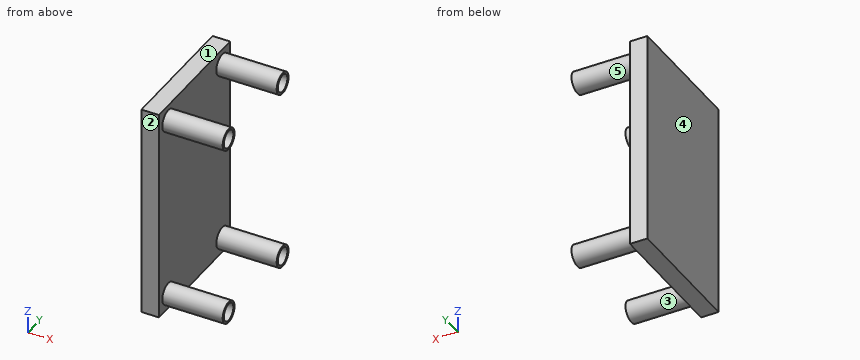
Autodesk Inventor part; units mm, degrees
ref_plane "YZ Plane" through (0, 0, 0) normal (1, 0, 0) x (0, 1, 0)
ref_plane "XZ Plane" through (0, 0, 0) normal (0, 1, 0) x (-1, 0, 0)
ref_plane "XY Plane" through (0, 0, 0) normal (0, 0, 1) x (1, 0, 0)
sketch "スケッチ1" plane through (0, 0, 0) normal (1, 0, 0) x (0, 1, 0)
  line L0 (13.9438, 85.4482) -> (-46.0562, 85.4482)
  line L1 (-46.0562, 85.4482) -> (-46.0562, -14.5518)
  line L2 (-46.0562, -14.5518) -> (13.9438, -14.5518)
  line L3 (13.9438, -14.5518) -> (13.9438, 85.4482)
  point P0 (0, 0)
  dimension "d0" = 60
  dimension "d1" = 100
extrude "押し出し1" add sketch "スケッチ1" along normal blind 8.1
sketch "スケッチ2" plane through (8.1, 0, 0) normal (1, 0, 0) x (0, 0, -1)
  circle A0 centre (-78.096, 7.3739) radius 5
  circle A1 centre (-78.096, -38.2101) radius 5
  circle A2 centre (7.3739, -38.2101) radius 5
  circle A3 centre (7.3739, 7.3739) radius 5
  circle A4 centre (-78.096, 7.3739) radius 4
  circle A5 centre (-78.096, -38.2101) radius 4
  circle A6 centre (7.3739, 7.3739) radius 4
  circle A7 centre (7.3739, -38.2101) radius 4
  point P0 (0, 0)
  dimension "d4" = 10
  dimension "d5" = 10
  dimension "d6" = 10
  dimension "d7" = 10
  dimension "d8" = 8
  dimension "d9" = 8
  dimension "d10" = 8
  dimension "d11" = 8
extrude "押し出し2" add sketch "スケッチ2" along normal blind 28
sketch "スケッチ3" plane through (0, 0, 0) normal (-1, 0, 0) x (0, 0, 1)
  point P0 (0, 0)
equation "\"BendRadius\" = Thickness"
equation "\"BendReliefWidth\" = Thickness"
equation "\"BendReliefDepth\" = 0.5 * Thickness"
equation "\"CornerReliefSize\" = 4 * Thickness"
equation "\"MinimumRemnant\" = 2 * Thickness"
equation "\"TransitionRadius\" = BendRadius"
equation "\"JacobiRadiusSize\" = BendRadius"
equation "\"GapSize\" = Thickness"
For this review, take the finished solid that the model builds, in its own axes (mm). Face numbers are marked on the shaded views. A direction names the side the tool comes from. Coordinates: 2 decimals unless noted, no trailing zeros. Write each loop counter-clockwise with the first axis right and the second up, starting at its lowest first coordinate (ties: lowest second). Pieces come first, ordered by that corner, then holes. Notation, with made-up numbers: (-20.5, 43.25) - (18.5, 43.25) arc R19 cw to (18.5, 56.25) - close; hole circle Ø4 at (23, 27). An arc over 180 degrees is marked (long way). Answer in a Markdown table with one row per item. Add a question column.
Q1. For probe 1 along Y at (x, z) = (33, 78.5); probe 2 along Y at (x, z) = (30, 81); probe 3 along Z at (x, y) = (33.5, -39), list the stretches that pass through material, from the lowest coordinate up.
Q2. We need section C-C, the plane z = -5. State the section outline as (x, y) points, and give its area (3 significant figures).
Q3. Tool access review of the marked faces 4 and 5: name each direction out of +Z, -Z, +X, -X, +Y, -Y from which nothing blocks a thin tool from reaching the whole face with its end or side.
Q4. Draft analysis for pull direction Y (two halves, no side actions). For the marked faces 1, 2 and 3, state which applies: +Y half, -Y half, draft (parallel to the pull), parting line (faces both ways), or undercut.
Q5. We need section D-D, the plane y = -40. State the section outline as (x, z) points.
Q6. We need section B-B, the plane y = -31.5. State the section outline as (x, z) points, and give its area (3 significant figures).
Q7. For P1, Ø1, axis at y = -35, z = 34, coming from the +X side; P2, Ø12, axis at x = 16.5, z = 12.5, coming from the -Y side; P3, Ø12, axis at x = 31.5, z = 3, coming from the +Y side, all flat-tipped, find the tip position at first contact; note any pin that passes through.
Q8. We need section A-A, the plane x = 22. State the section outline as (y, z) points, and give its area (3 significant figures).
Answer list:
| question | item | result |
|---|---|---|
| 1 | probe 1 | y = -43.19 to -42.19, -34.23 to -33.23, 2.39 to 3.39, 11.35 to 12.36 |
| 1 | probe 2 | y = -42.28 to -40.96, -35.46 to -34.14, 3.3 to 4.62, 10.12 to 11.44 |
| 1 | probe 3 | z = -12.31 to -11.3, -3.45 to -2.44, 73.16 to 74.17, 82.02 to 83.03 |
| 2 | outline | (0, -46.06) - (8.1, -46.06) - (8.1, -42.61) - (36.1, -42.61) - (36.1, -41.43) - (8.1, -41.43) - (8.1, -34.99) - (36.1, -34.99) - (36.1, -33.81) - (8.1, -33.81) - (8.1, 2.97) - (36.1, 2.97) - (36.1, 4.15) - (8.1, 4.15) - (8.1, 10.59) - (36.1, 10.59) - (36.1, 11.77) - (8.1, 11.77) - (8.1, 13.94) - (0, 13.94) - close |
| 2 | area | 618 mm2 |
| 3 | face 4 | +Z, -Z, -X, +Y, -Y |
| 3 | face 5 | +X |
| 4 | face 1 | draft |
| 4 | face 2 | -Y half |
| 4 | face 3 | undercut |
| 5 | outline | (0, -14.55) - (8.1, -14.55) - (8.1, -12.04) - (36.1, -12.04) - (36.1, -10.95) - (8.1, -10.95) - (8.1, -3.8) - (36.1, -3.8) - (36.1, -2.71) - (8.1, -2.71) - (8.1, 73.43) - (36.1, 73.43) - (36.1, 74.52) - (8.1, 74.52) - (8.1, 81.67) - (36.1, 81.67) - (36.1, 82.76) - (8.1, 82.76) - (8.1, 85.45) - (0, 85.45) - close |
| 6 | outline | (0, -14.55) - (8.1, -14.55) - (8.1, 85.45) - (0, 85.45) - close |
| 6 | area | 810 mm2 |
| 7 | P1 | stops at x = 8.1 |
| 7 | P2 | passes through |
| 7 | P3 | stops at y = 9.8 |
| 8 | outline | circle Ø10 at (-38.21, -7.37); circle Ø10 at (-38.21, 78.1); circle Ø10 at (7.37, -7.37); circle Ø10 at (7.37, 78.1); hole circle Ø8 at (-38.21, -7.37); hole circle Ø8 at (-38.21, 78.1); hole circle Ø8 at (7.37, -7.37); hole circle Ø8 at (7.37, 78.1) |
| 8 | area | 113 mm2 |
